The model under review builds one solid part; all positions refer to its coordinate system, in mm. A direction names the side the tool comes from. Round coordinates to 2 decimals unless told otherwise and drop trailing zeros. Order: outer loops, then holes, each group sorted by start corner. A loop starts at its lowest first (then second) coordinate and runs counter-clockwise, first axis right, second up. Notation, with made-up numbers: M 58.25,44 L 75.25,44 A12 cw 75.25,50 Z; hole C 52,15 d11. An arc over 180 degrees is marked long. Answer as CSV lines item,"result". Start each with the question number.
from build123d import *

# Parameters (mm, degrees)
BOSS_EXTRUDE1_DEPTH = 6


with BuildPart() as part:
    # Sketch1 → Boss-Extrude1 (new body)
    with BuildSketch(Plane.XY):
        Polygon((57.521474666, -355.462944523), (44.521477546, -368.462941643), (44.521477546, -387.422916834), (57.521474666, -400.462926923), (78.921469418, -400.462926923), (78.921469418, -394.222907142), (83.271467309, -394.222907142), (83.7891054, -394.154758794), (84.271467309, -393.954957949), (84.685680872, -393.637120704), (85.003518117, -393.222907142), (85.203318962, -392.740545232), (85.271467309, -392.222907142), (85.271467309, -387.422911176), (85.203318962, -386.905273086), (85.003518117, -386.422911176), (84.685680872, -386.008697614), (84.271467309, -385.690860369), (83.7891054, -385.491059524), (83.271467309, -385.422911176), (78.921469418, -385.422911176), (78.921469418, -380.12291917), (73.621470596, -380.12291917), (73.621470596, -381.922917402), (68.521472832, -381.922917402), (68.521472832, -380.12291917), (64.57147301, -380.12291917), (64.57147301, -375.722914498), (68.521472832, -375.722914498), (68.521472832, -373.922916266), (73.621470596, -373.922916266), (73.621470596, -375.722914498), (78.921469418, -375.722914498), (78.921469418, -370.422917243), (83.271467309, -370.422917243), (83.7891054, -370.354768896), (84.271467309, -370.154968051), (84.685680872, -369.837130805), (85.003518117, -369.422917243), (85.203318962, -368.940555333), (85.271467309, -368.422917243), (85.271467309, -363.622922801), (85.203318962, -363.105284711), (85.003518117, -362.622922801), (84.685680872, -362.208709239), (84.271467309, -361.890871993), (83.7891054, -361.691071148), (83.271467309, -361.622922801), (78.921469418, -361.622922801), (78.921469418, -355.462944523), align=None)
        Polygon((50.398749784, -377.922916834), (50.535046479, -378.958193014), (50.934648169, -379.922916834), (51.57032266, -380.751343959), (52.398749784, -381.387018449), (53.363473604, -381.786620139), (54.398749784, -381.922916834), (55.434025965, -381.786620139), (56.398749784, -381.387018449), (57.227176909, -380.751343959), (57.862851399, -379.922916834), (58.262453089, -378.958193014), (58.398749784, -377.922916834), (58.262453089, -376.887640653), (57.862851399, -375.922916834), (57.227176909, -375.094489709), (56.398749784, -374.458815219), (55.434025965, -374.059213529), (54.398749784, -373.922916834), (53.363473604, -374.059213529), (52.398749784, -374.458815219), (51.57032266, -375.094489709), (50.934648169, -375.922916834), (50.535046479, -376.887640653), align=None, mode=Mode.SUBTRACT)
    extrude(amount=BOSS_EXTRUDE1_DEPTH)


solid = part.part
Item 1: For pin 1 (2 mm diameter, centred on y = -377, z = 2.5, fed in from +X); pin 2 (10 mm diameter, centred on x = 72.5, y = -370, fed in from -Z); pin 3 (2 mm diameter, centred on x = 80, z = 3, fed in from -Y); pin 4 (1.5 mm diameter, centred on x = 55.5, z = 3, fed in from -Y), all flat-tipped, find the tip position at first contact; note any pin that passes through.
Item 2: Tool access review of faces 4 (the flat face through (81, -394.223, 3)), 5 (the flat face through (85.271, -390, 3)), 6 (the flat face through (76, -375.723, 3)), 7 (the flat face through (73.621, -381, 3)), 8 (the flat face through (68, -400.463, 3)): name each direction out of +Z, -Z, +X, -X, +Y, -Y from which nothing blocks a thin tool from reaching the whole face with its end or side.
Item 3: Consider section A-A (x = 72). State the section outline as (y, z) points.
Item 4: Wall thickness on probe 1 along Y at (x, z) = (82, 3.8); probe 2 along Y at (x, z) = (72, 1.5); probe 3 along X at (y, z) = (-387, 0.3): over which ranges is each line inside the solid? List them lowest first. Write a range as [from, to].
Item 5: Consider section C-C (y = -367). State the section outline as (x, z) points.
Item 6: Consider section B-B (y = -359). State the section outline as (x, z) points, and give its area (3 significant figures).
Item 7: The part is to be moulded in two halves that separate along X. For faces 1 (the flat face through (78.921, -373, 3)), 2 (the flat face through (50.466, -378.433, 2.958)), 3 (the flat face through (44.521, -378, 3)), say which applies: +X half, -X half, draft (parallel to the pull), parting line (faces both ways), or undercut.
Reported:
1,pin 1,"stops at x = 64.57"
1,pin 2,"stops at z = 0"
1,pin 3,"stops at y = -394.22"
1,pin 4,"stops at y = -399.19"
2,face 4,"+Z, -Z, +X, -Y"
2,face 5,"+Z, -Z, +X, +Y, -Y"
2,face 6,"+Z, -Z, +X"
2,face 7,"+Z, -Z"
2,face 8,"+Z, -Z, +X, -X, -Y"
3,outline,"M -400.46,0 L -381.92,0 L -381.92,6 L -400.46,6 Z; M -373.92,0 L -355.46,0 L -355.46,6 L -373.92,6 Z"
4,probe 1,"y = [-394.22, -385.42], [-370.42, -361.62]"
4,probe 2,"y = [-400.46, -381.92], [-373.92, -355.46]"
4,probe 3,"x = [44.52, 85.22]"
5,outline,"M 45.98,0 L 85.27,0 L 85.27,6 L 45.98,6 Z"
6,outline,"M 53.98,0 L 78.92,0 L 78.92,6 L 53.98,6 Z"
6,area,"150 mm²"
7,face 1,"+X half"
7,face 2,"undercut"
7,face 3,"-X half"
